Geometry: final body of the model. Coordinates: model frame, mm. A direction names the side the tool comes from. Coordinates: 2 decimals unless noted, no trailing zeros. Write each loop counter-clockwise with the first axis right and the second up, starting at its lowest first coordinate (ties: lowest second). Pieces come first, ordered by that corner, then holes.
from build123d import *

# Parameters (mm, degrees)
SKETCH_1_R      = 1.65
SKETCH_1_R_2    = 10
SKETCH_1_R_3    = 8.25
EXTRUDE_1_DEPTH = 3
SKETCH_1_3_R    = 8.25
EXTRUDE_2_DEPTH = 2


with BuildPart() as part:
    # Sketch 1 → Extrude 1 (new body)
    # profile 1 of 3: a face of its own
    with BuildSketch(Plane.XY):
        with BuildLine():
            Line((-4.615384615, 14.923076923), (-9.230769231, 3.846153846))
            ThreePointArc((-9.230769231, 3.846153846), (0, 10), (9.230769231, 3.846153846))
            Line((9.230769231, 3.846153846), (4.615384615, 14.923076923))
            ThreePointArc((4.615384615, 14.923076923), (0, 18), (-4.615384615, 14.923076923))
        make_face()
        with Locations((0, 13)):
            Circle(SKETCH_1_R, mode=Mode.SUBTRACT)
    # profile 2 of 3: a face of its own
    with BuildSketch(Plane.XY):
        Circle(SKETCH_1_R_2)
        Circle(SKETCH_1_R_3, mode=Mode.SUBTRACT)
    # profile 3 of 3: a face of its own
    with BuildSketch(Plane.XY):
        with BuildLine():
            ThreePointArc((9.230769231, -3.846153846), (0, -10), (-9.230769231, -3.846153846))
            Line((-9.230769231, -3.846153846), (-4.615384615, -14.923076923))
            ThreePointArc((-4.615384615, -14.923076923), (0, -18), (4.615384615, -14.923076923))
            Line((4.615384615, -14.923076923), (9.230769231, -3.846153846))
        make_face()
        with Locations((0, -13)):
            Circle(SKETCH_1_R, mode=Mode.SUBTRACT)
    extrude(amount=EXTRUDE_1_DEPTH)

    # Sketch 1_3 → Extrude 2 (add)
    with BuildSketch(Plane.XY):
        Circle(SKETCH_1_3_R)
    extrude(amount=EXTRUDE_2_DEPTH)


solid = part.part
Item 1: Material intervals for probe 1 along Y at (x, z) = (0, 0.65); probe 2 along Y at (x, z) = (0, 2.8); probe 3 along Y at (x, z) = (-1.5, 2.8), sorted ascending.
Derived:
probe 1: y = -18 to -14.65, -11.35 to 11.35, 14.65 to 18
probe 2: y = -18 to -14.65, -11.35 to -8.25, 8.25 to 11.35, 14.65 to 18
probe 3: y = -17.77 to -13.69, -12.31 to -8.11, 8.11 to 12.31, 13.69 to 17.77
Item 2: Pull-direction query (Y, two-part tool) for faces 3 (the cylindrical face through (7.62, -3.16, 2.49)), 4 (the flat face through (6.89, -9.46, 1.48)), 5 (the flat face through (-2.4, 8.3, 3)); classes: released by +Y, released by -Y, zero draft, split by the parting line, or undercut.
Derived:
face 3: undercut
face 4: released by -Y
face 5: zero draft
Item 3: Set-up query: faces 1 (the cylindrical face through (10, 0, 1)), 2 (the flat face through (0, 0, 2)). Return all of +Z, -Z, +X, -X, +Y, -Y with unobstructed straight access to the full face (end or side cutting, diameter ignored); none if empty.
Derived:
face 1: +Z, -Z, +X
face 2: +Z
Item 4: Pin query (flat end, axial travel): pin 1 (8 mm diameter, centred on x = -3, y = -2.5, fed in from +Z). Return the tip coordinate at first contact, or that it passes through.
Derived:
pin 1: stops at z = 2
Item 5: Section B-B, the plane y = 13.5. Output: boundary loops of the cut face in (x, z).
Derived:
outline: (-5.21, 0) - (-1.57, 0) - (-1.57, 3) - (-5.21, 3) - close; (1.57, 0) - (5.21, 0) - (5.21, 3) - (1.57, 3) - close
Item 6: Section A-A, the plane x = 0. Output: boundary loops of the cut face in (y, z).
Derived:
outline: (-18, 0) - (-14.65, 0) - (-14.65, 3) - (-18, 3) - close; (-11.35, 0) - (11.35, 0) - (11.35, 3) - (8.25, 3) - (8.25, 2) - (-8.25, 2) - (-8.25, 3) - (-11.35, 3) - close; (14.65, 0) - (18, 0) - (18, 3) - (14.65, 3) - close
Item 7: Section C-C, the plane z = 0.4. Output: boundary loops of the cut face in (x, y), plus the area to 3 significant figures.
Derived:
outline: (-9.23, -3.85) - (-4.62, -14.92) arc R5 ccw to (4.62, -14.92) - (9.23, -3.85) arc R10 ccw to (9.23, 3.85) - (4.62, 14.92) arc R5 ccw to (-4.62, 14.92) - (-9.23, 3.85) arc R10 ccw to start; hole circle Ø3.3 at (0, -13); hole circle Ø3.3 at (0, 13)
area: 481 mm2
Item 8: Section D-D, the plane y = 0. Output: boundary loops of the cut face in (x, z), plus the area to 3 significant figures.
Derived:
outline: (-10, 0) - (10, 0) - (10, 3) - (8.25, 3) - (8.25, 2) - (-8.25, 2) - (-8.25, 3) - (-10, 3) - close
area: 43.5 mm2
